Check sheet for the modelled part. Datum: model origin and axes. Units: mm. Face numbers are marked on the shaded views. Coordinates: 2 decimals unless noted, no trailing zeros. Write each loop counter-clockwise with the first axis right and the second up, starting at its lowest first coordinate (ties: lowest second). Pieces come first, ordered by that corner, then holes. Notation, with made-up numbers: (45, 42.25) -> (50, 42.25) arc R34 cw to (50, 80.25) -> close; hole circle Ø10 at (-32, 42.25). An arc over 180 degrees is marked (long way). Put each result on its own line as item: value.
```python
from build123d import *

# Parameters (mm, degrees)
EXTRUDE_1_DEPTH = 3


with BuildPart() as part:
    # 草图1 → 凸台-拉伸1 (new body)
    with BuildSketch(Plane(origin=(0, 0, 0), x_dir=(1, 0, 0), z_dir=(0, 1, 0))):
        with BuildLine():
            Line((-15, 17.5), (15, 17.5))
            ThreePointArc((15, 17.5), (18.535533906, 16.035533906), (20, 12.5))
            Line((20, 12.5), (20, -12.5))
            ThreePointArc((20, -12.5), (18.535533906, -16.035533906), (15, -17.5))
            Line((15, -17.5), (-15, -17.5))
            ThreePointArc((-15, -17.5), (-18.535533906, -16.035533906), (-20, -12.5))
            Line((-20, -12.5), (-20, 12.5))
            ThreePointArc((-20, 12.5), (-18.535533906, 16.035533906), (-15, 17.5))
        make_face()
        with BuildLine():
            Line((5, -11), (15, -11))
            ThreePointArc((15, -11), (16.5, -12.5), (15, -14))
            Line((15, -14), (5, -14))
            ThreePointArc((5, -14), (3.5, -12.5), (5, -11))
        make_face(mode=Mode.SUBTRACT)
        with BuildLine():
            Line((-15, -14), (-5, -14))
            ThreePointArc((-5, -14), (-3.5, -12.5), (-5, -11))
            Line((-5, -11), (-15, -11))
            ThreePointArc((-15, -11), (-16.5, -12.5), (-15, -14))
        make_face(mode=Mode.SUBTRACT)
        with BuildLine():
            Line((-14.869936395, -1.121838378), (-4.869936395, -1.121838378))
            ThreePointArc((-4.869936395, -1.121838378), (-3.369936395, -2.621838378), (-4.869936395, -4.121838378))
            Line((-4.869936395, -4.121838378), (-14.869936395, -4.121838378))
            ThreePointArc((-14.869936395, -4.121838378), (-16.369936395, -2.621838378), (-14.869936395, -1.121838378))
        make_face(mode=Mode.SUBTRACT)
        with BuildLine():
            Line((4.869936395, -4.121838378), (14.869936395, -4.121838378))
            ThreePointArc((14.869936395, -4.121838378), (16.369936395, -2.621838378), (14.869936395, -1.121838378))
            Line((14.869936395, -1.121838378), (4.869936395, -1.121838378))
            ThreePointArc((4.869936395, -1.121838378), (3.369936395, -2.621838378), (4.869936395, -4.121838378))
        make_face(mode=Mode.SUBTRACT)
        with BuildLine():
            Line((-1.5, 12.5), (-1.5, 0))
            ThreePointArc((-1.5, 0), (0, -1.5), (1.5, 0))
            Line((1.5, 0), (1.5, 12.5))
            ThreePointArc((1.5, 12.5), (0, 14), (-1.5, 12.5))
        make_face(mode=Mode.SUBTRACT)
    extrude(amount=EXTRUDE_1_DEPTH)


solid = part.part
```
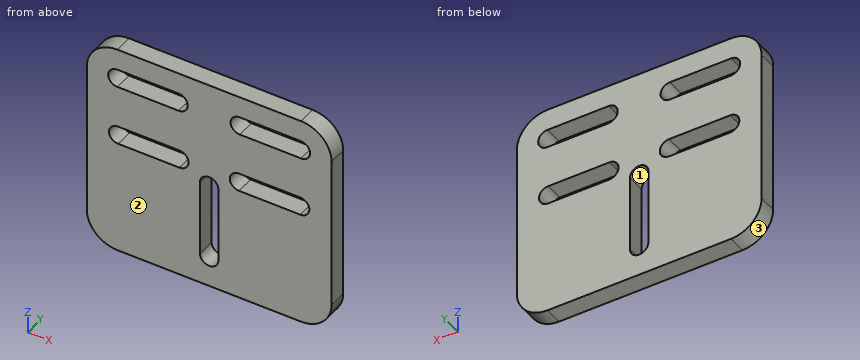
Q1. Cross-section at D-D (y = 1.05). Record the cut outline in (x, z), plus the area to 3 significant figures.
Recorded:
outline: (-20, -12.5) arc R5 ccw to (-15, -17.5) -> (15, -17.5) arc R5 ccw to (20, -12.5) -> (20, 12.5) arc R5 ccw to (15, 17.5) -> (-15, 17.5) arc R5 ccw to (-20, 12.5) -> close; hole (-15, 11) -> (-5, 11) arc R1.5 ccw to (-5, 14) -> (-15, 14) arc R1.5 ccw to start; hole (-14.87, 1.12) -> (-4.87, 1.12) arc R1.5 ccw to (-4.87, 4.12) -> (-14.87, 4.12) arc R1.5 ccw to start; hole (-1.5, -12.5) arc R1.5 ccw to (1.5, -12.5) -> (1.5, 0) arc R1.5 ccw to (-1.5, 0) -> close; hole (4.87, 1.12) -> (14.87, 1.12) arc R1.5 ccw to (14.87, 4.12) -> (4.87, 4.12) arc R1.5 ccw to start; hole (5, 11) -> (15, 11) arc R1.5 ccw to (15, 14) -> (5, 14) arc R1.5 ccw to start
area: 1,190 mm2
Q2. Cross-section at B-B (x = 9). Record the cut outline in (y, z), plus the area to 3 significant figures.
Recorded:
outline: (0, -17.5) -> (3, -17.5) -> (3, 1.12) -> (0, 1.12) -> close; (0, 4.12) -> (3, 4.12) -> (3, 11) -> (0, 11) -> close; (0, 14) -> (3, 14) -> (3, 17.5) -> (0, 17.5) -> close
area: 87.0 mm2
Q3. Cross-section at A-A (x = 0). Record the cut outline in (y, z).
Recorded:
outline: (0, -17.5) -> (3, -17.5) -> (3, -14) -> (0, -14) -> close; (0, 1.5) -> (3, 1.5) -> (3, 17.5) -> (0, 17.5) -> close
Q4. Cross-section at C-C (z = 2). Record the cut outline in (x, y).
Recorded:
outline: (-20, 0) -> (-16.23, 0) -> (-16.23, 3) -> (-20, 3) -> close; (-3.5, 0) -> (3.5, 0) -> (3.5, 3) -> (-3.5, 3) -> close; (16.23, 0) -> (20, 0) -> (20, 3) -> (16.23, 3) -> close
Q5. Mould release check, pull along Z, two halves, no side actions. Record for the marked faces 1, 2 and 3: released by +Z, released by -Z, zero draft, split by the parting line, or undercut.
Recorded:
face 1: undercut
face 2: zero draft
face 3: released by -Z
Q6. Material ranges on line 1 along Z through (x, y) = (-12.5, 2); line 2 along X through (y, z) = (0.15, 2.5); line 3 along X through (y, z) = (0.2, -9), recorded low to high.
Recorded:
line 1: z = -17.5 to 1.12, 4.12 to 11, 14 to 17.5
line 2: x = -20 to -16.36, -3.37 to 3.37, 16.36 to 20
line 3: x = -20 to -1.5, 1.5 to 20
